Could you check a few things on this model? Use its own coordinates, in mm. Face numbers are marked on the shaded views. A direction names the side the tool comes from. Round coordinates to 2 decimals unless told otherwise and drop trailing zeros. Order: outer loops, then holes, each group sorted by start corner. A loop starts at its lowest first (then second) coordinate and runs counter-clockwise, first axis right, second up. Notation, with made-up numbers: (11.25, 43.25) - (20.25, 43.25) arc R32 cw to (20.25, 74.25) - close; hole circle Ø8 at (62, 86). An arc over 180 degrees is marked (long way). Use one line per item in the form item = value.
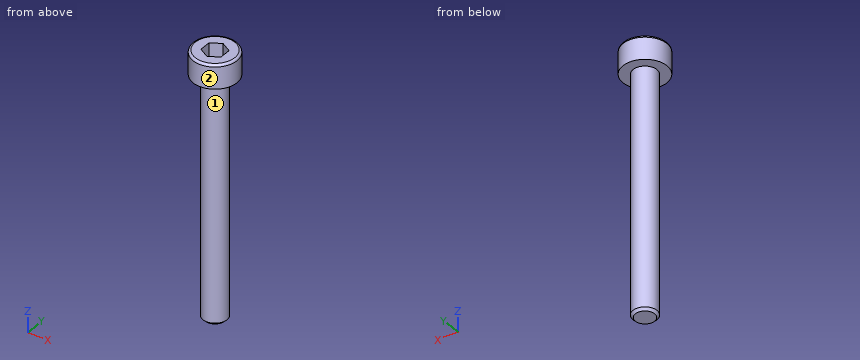
from build123d import *

# Parameters (mm, degrees)
CUT_EXTRUDE_1_DEPTH = 1.925
FILLET_1_R          = 0.275
CHAMFER_1_SIZE      = 0.3


with BuildPart() as part:
    # 草图3 → 旋转1 (revolve)
    with BuildSketch(Plane(origin=(0, 0, 0), x_dir=(0, 0, -1), z_dir=(1, 0, 0)), mode=Mode.PRIVATE) as revolve_1_sk:
        Polygon((-3, 0), (-3, 2.75), (0, 2.75), (0, 1.5), (30, 1.5), (30, 0), align=None)
    revolve(revolve_1_sk.sketch.rotate(Axis((0, 0, 3), (0, 0, -1)), 180), axis=Axis((0, 0, 3), (0, 0, -1)))

    # 草图4 → 切除-拉伸1 (cut)
    with BuildSketch(Plane.XY.offset(3)):
        Polygon((0, 1.443375673), (-1.25, 0.721687836), (-1.25, -0.721687836), (0, -1.443375673), (1.25, -0.721687836), (1.25, 0.721687836), align=None)
    extrude(amount=-CUT_EXTRUDE_1_DEPTH, mode=Mode.SUBTRACT)

    # 圆角1
    fillet_1_edges = [part.edges().sort_by_distance(p)[0] for p in [
        (0, 2.75, 3),
    ]]
    fillet(fillet_1_edges, radius=FILLET_1_R)

    # 倒角1
    chamfer_1_edges = [part.edges().sort_by_distance(p)[0] for p in [
        (0, 1.5, -30),
    ]]
    chamfer(chamfer_1_edges, length=CHAMFER_1_SIZE)


solid = part.part
Item 1: I need wall thicknesses on L1, parallel to Z at x = 1.95, y = 1.3; L2, parallel to X at y = 0.4, z = -15; L3, parallel to X at y = -0.15, z = -14.5. Which ranges of each line are inside material? Lowest first, please.
Found:
L1 = 0 to 3
L2 = -1.45 to 1.45
L3 = -1.49 to 1.49
Item 2: Imagine slicing it at B-B on z = -19.5. Please give me the cut outline in (x, y), plus the area to 3 significant figures.
Found:
outline = circle Ø3 at (0, 0)
area = 7.07 mm2
Item 3: Will these pins go through, and if not, where does the flat tip stop? P1, Ø3, axis at x = -1, z = -6.5, coming from the -Y side; P2, Ø1, axis at x = -1, z = -24, coming from the -Y side.
Found:
P1 = -1.5
P2 = -1.41
Item 4: For the marked faces 1 and 2, which set-ups out of +Z, -Z, +X, -X, +Y, -Y let a thin tool reach every point of the face, with its end or its side?
Found:
face_1 = -Z
face_2 = +Z, -Z
Item 5: Imagine slicing it at A-A on y = 0. Please give me the cut outline in (x, z) (3 decimals), plus the area to 3 significant figures.
Found:
outline = (-2.75, 0) - (-1.5, 0) - (-1.5, -29.7) - (-1.2, -30) - (1.2, -30) - (1.5, -29.7) - (1.5, 0) - (2.75, 0) - (2.75, 2.725) arc R0.275 ccw to (2.475, 3) - (1.25, 3) - (1.25, 1.075) - (-1.25, 1.075) - (-1.25, 3) - (-2.475, 3) arc R0.275 ccw to (-2.75, 2.725) - close
area = 102 mm2
